from build123d import *

# Parameters (mm, degrees)
F1_W     = 5
F1_H     = 7.2
F1_H_2   = 6
F1_H_3   = 4
F1_W_2   = 23.3
F3_DEPTH = 8.5
F0_W     = 23.3
F0_H     = 4
F4_DEPTH = 23.2
F5_DEPTH = 18.1
F6_START = 4.3
F0_R     = 0.85
F6_DEPTH = 20.7


with BuildPart() as f3:
    # F1 (on Front) → F3 (new body, symmetric)
    with BuildSketch(Plane.XZ):
        with Locations((-14.15, 13.6)):
            Rectangle(F1_W, F1_H)
        with Locations((-14.15, 20.2)):
            Rectangle(F1_W, F1_H_2)
        with Locations((-14.15, 7)):
            Rectangle(F1_W, F1_H_2)
        with Locations((-14.15, 2)):
            Rectangle(F1_W, F1_H_3)
        with Locations((0, 2)):
            Rectangle(F1_W_2, F1_H_3)
        with Locations((14.15, 2)):
            Rectangle(F1_W, F1_H_3)
        with Locations((14.15, 7)):
            Rectangle(F1_W, F1_H_2)
        with Locations((14.15, 13.6)):
            Rectangle(F1_W, F1_H)
        with Locations((14.15, 20.2)):
            Rectangle(F1_W, F1_H_2)
    extrude(amount=F3_DEPTH, both=True)

    # F0 (on Top) → F4 (join)
    with BuildSketch(Plane.XY):
        with Locations((0, 6.5)):
            Rectangle(F0_W, F0_H)
    extrude(amount=F4_DEPTH)

    # F2 (on Right) → F5 (cut, symmetric)
    with BuildSketch(Plane.YZ):
        with BuildLine():
            Line((-8.5, 17.2), (-8.5, 10))
            Line((-8.5, 10), (3.5396314061, 10))
            ThreePointArc((3.5396314061, 10), (2.8089650426, 10.8020152096), (1.9224991399, 11.4275389379))
            Line((1.9224991399, 11.4275389379), (-5.9224991399, 15.7724610621))
            ThreePointArc((-5.9224991399, 15.7724610621), (-6.8089650426, 16.3979847904), (-7.5396314061, 17.2))
            Line((-7.5396314061, 17.2), (-8.5, 17.2))
        make_face()
        with BuildLine():
            Line((-8.5, 20.1464178425), (-8.5, 17.2))
            Line((-8.5, 17.2), (-7.5396314061, 17.2))
            ThreePointArc((-7.5396314061, 17.2), (-8.2538488107, 18.5969271247), (-8.5, 20.1464178425))
        make_face()
        with BuildLine():
            Line((-8.5, 10), (-8.5, 4))
            Line((-8.5, 4), (4.5, 4))
            Line((4.5, 4), (4.5, 7.0535821575))
            ThreePointArc((4.5, 7.0535821575), (4.2538488107, 8.6030728753), (3.5396314061, 10))
            Line((3.5396314061, 10), (-8.5, 10))
        make_face()
    extrude(amount=F5_DEPTH, both=True, mode=Mode.SUBTRACT)

    # F0 (on Top) → F6 (cut)
    with BuildSketch(Plane.XY.offset(F6_START)):
        with Locations((14.15, -2)):
            Circle(F0_R)
        with Locations((-14.15, -2)):
            Circle(F0_R)
    extrude(amount=F6_DEPTH, mode=Mode.SUBTRACT)


solid = f3.part
Design review of the part built by this model. Coordinates are the model's own, in mm. A direction names the side the tool comes from. Round coordinates to 2 decimals unless told otherwise and drop trailing zeros. Write each loop counter-clockwise with the first axis right and the second up, starting at its lowest first coordinate (ties: lowest second). Pieces come first, ordered by that corner, then holes. Notation, with made-up numbers: M 76.25,87 L 134.25,87 A19 ccw 134.25,100 Z; hole C 84.5,48 d10. An arc over 180 degrees is marked long. One line per item, written item: value. Start each with the question number.
1. To check wall thickness, follow probe 1 along X at (y, z) = (-2, 20); probe 2 along Y at (x, z) = (14.15, 21); probe 3 along X at (y, z) = (1, 22). State the ranges of each line that lie inside material, in increasing order. Write a range as from..to.
2. Clearance check with flat-ended pins moving along their axes: P1, Ø1.5, axis at x = -14.15, y = -2, coming from the +Z side; P2, Ø8, axis at x = -2.5, z = 15, coming from the -Y side; P3, Ø1, axis at y = -1.5, z = 11, coming from the +X side. State where each tip first meets the part, or that it passes through.
3. Take a section at A-A on y = -2. State the section outline as (x, z) points.
4. Take a section at D-D on y = -6.75. State the section outline as (x, z) points.
5. Take a section at B-B on x = -14. State the section outline as (y, z) points.
6. Take a section at C-C on z = 16.25. State the section outline as (x, y) points, then the cut area to 3 significant figures.
7. Draft analysis for pull direction Y (two halves, no side actions). For faces 1 (the face through (0, 4.5, 13)), 2 (the face through (-13.693, -1.283, 18.046)), 3 (the face through (-16.65, 2, 14)), state which applies: pulls with the +Y half, pulls with the -Y half, needs draft (parallel to the pull), parting line crosses it, or undercut.
8. For faces 4 (the face through (14.039, -1.157, 18.046)), 5 (the face through (13.074, -1.945, 13.57)), 6 (the face through (11.65, -1, 19)), list the 3-axis set-ups (+Z, -Z, +X, -X, +Y, -Y) from which the entire face can be reached by the end or side of a thin tool; tool diameter is ignored.
Computed:
1. probe 1: x = -16.65..-15, -13.3..-11.65, 11.65..13.3, 15..16.65
1. probe 2: y = -8.5..-2.85, -1.15..8.5
1. probe 3: x = -16.65..-11.65, 11.65..16.65
2. P1: stops at z = 4
2. P2: stops at y = 4.5
2. P3: passes through
3. outline: M -16.65,0 L 16.65,0 L 16.65,4 L -16.65,4 Z; M -16.65,13.6 L -15,13.6 L -15,23.2 L -16.65,23.2 Z; M -13.3,13.6 L -11.65,13.6 L -11.65,23.2 L -13.3,23.2 Z; M 11.65,13.6 L 13.3,13.6 L 13.3,23.2 L 11.65,23.2 Z; M 15,13.6 L 16.65,13.6 L 16.65,23.2 L 15,23.2 Z
4. outline: M -16.65,0 L 16.65,0 L 16.65,4 L -16.65,4 Z; M -16.65,16.35 L -11.65,16.35 L -11.65,23.2 L -16.65,23.2 Z; M 11.65,16.35 L 16.65,16.35 L 16.65,23.2 L 11.65,23.2 Z
5. outline: M -8.5,0 L 8.5,0 L 8.5,23.2 L -1.16,23.2 L -1.16,13.14 L 1.92,11.43 A5 cw 4.5,7.05 L 4.5,4 L -8.5,4 Z; M -8.5,20.15 A5 ccw -5.92,15.77 L -2.84,14.06 L -2.84,23.2 L -8.5,23.2 Z
6. outline: M -16.65,-6.63 L -11.65,-6.63 L -11.65,4.5 L 11.65,4.5 L 11.65,-6.63 L 16.65,-6.63 L 16.65,8.5 L -16.65,8.5 Z; hole C -14.15,-2 d1.7; hole C 14.15,-2 d1.7
6. area: 240 mm²
7. face 1: pulls with the -Y half
7. face 2: undercut
7. face 3: needs draft
8. face 4: +Z
8. face 5: +X, -X, -Y
8. face 6: +Z, -Y
